Here's how the part is built. I have some questions about the finished solid (model axes, mm). A direction names the side the tool comes from. Give positions to 0.01 mm unless a question says otherwise; leave off trailing zeros. Order: outer loops, then holes, each group sorted by start corner. A loop starts at its lowest first (then second) coordinate and runs counter-clockwise, first axis right, second up.
from build123d import *

# Parameters (mm, degrees)
SKETCH_1_R      = 1.6
SKETCH_1_R_2    = 8
SKETCH_1_R_3    = 7.1
EXTRUDE_1_DEPTH = 5
SKETCH_1_3_R    = 7.1
SKETCH_1_3_R_2  = 2.1
EXTRUDE_2_DEPTH = 3
FILLET_1_R      = 1
FILLET_2_R      = 1
FILLET_3_R      = 1
FILLET_4_R      = 1


with BuildPart() as part:
    # Sketch 1 → Extrude 1 (new body)
    with BuildSketch(Plane(origin=(0, 0, 0), x_dir=(1, 0, 0), z_dir=(0, 1, 0))):
        with BuildLine():
            Line((1.92, -15.884382267), (51.2, -9.927738917))
            ThreePointArc((51.2, -9.927738917), (60, 0), (51.2, 9.927738917))
            Line((51.2, 9.927738917), (1.92, 15.884382267))
            ThreePointArc((1.92, 15.884382267), (-16, 0), (1.92, -15.884382267))
        make_face()
        with Locations((-12, 0)):
            Circle(SKETCH_1_R, mode=Mode.SUBTRACT)
        with Locations((0, 12)):
            Circle(SKETCH_1_R, mode=Mode.SUBTRACT)
        with Locations((12, 0)):
            Circle(SKETCH_1_R, mode=Mode.SUBTRACT)
        with Locations((0, -12)):
            Circle(SKETCH_1_R, mode=Mode.SUBTRACT)
        Circle(SKETCH_1_R_2, mode=Mode.SUBTRACT)
        with Locations((50, 0)):
            Circle(SKETCH_1_R_3, mode=Mode.SUBTRACT)
        Polygon((18.356508588, 8.861251331), (38.535462938, 6.422151611), (30.734984007, 2.266153232), align=None, mode=Mode.SUBTRACT)
        Polygon((18.356508588, -8.861251331), (38.535462938, -6.422151611), (30.734984007, -2.266153232), align=None, mode=Mode.SUBTRACT)
        with BuildLine():
            Line((14.72234722, 6.265180949), (26.481594346, 0))
            Line((26.481594346, 0), (14.72234722, -6.265180949))
            ThreePointArc((14.72234722, -6.265180949), (16, 0), (14.72234722, 6.265180949))
        make_face(mode=Mode.SUBTRACT)
        with BuildLine():
            Line((34.988373668, 0), (40.429404433, -2.898913674))
            ThreePointArc((40.429404433, -2.898913674), (40, 0), (40.429404433, 2.898913674))
            Line((40.429404433, 2.898913674), (34.988373668, 0))
        make_face(mode=Mode.SUBTRACT)
    extrude(amount=EXTRUDE_1_DEPTH)

    # Sketch 1_3 → Extrude 2 (add)
    with BuildSketch(Plane(origin=(0, 0, 0), x_dir=(1, 0, 0), z_dir=(0, 1, 0))):
        with Locations((50, 0)):
            Circle(SKETCH_1_3_R)
        with Locations((50, 0)):
            Circle(SKETCH_1_3_R_2, mode=Mode.SUBTRACT)
    extrude(amount=EXTRUDE_2_DEPTH)

    # Fillet 1
    fillet_1_edges = [part.edges().sort_by_distance(p)[0] for p in [
        (34.988373668, 2.5, 0),
        (40.429404433, 2.5, 2.898913674),
        (40.429404433, 2.5, -2.898913674),
    ]]
    fillet(fillet_1_edges, radius=FILLET_1_R)

    # Fillet 2
    fillet_2_edges = [part.edges().sort_by_distance(p)[0] for p in [
        (18.356508588, 2.5, 8.861251331),
        (38.535462938, 2.5, 6.422151611),
        (30.734984007, 2.5, 2.266153232),
    ]]
    fillet(fillet_2_edges, radius=FILLET_2_R)

    # Fillet 3
    fillet_3_edges = [part.edges().sort_by_distance(p)[0] for p in [
        (38.535462938, 2.5, -6.422151611),
        (18.356508588, 2.5, -8.861251331),
        (30.734984007, 2.5, -2.266153232),
    ]]
    fillet(fillet_3_edges, radius=FILLET_3_R)

    # Fillet 4
    fillet_4_edges = [part.edges().sort_by_distance(p)[0] for p in [
        (26.481594346, 2.5, 0),
        (14.72234722, 2.5, -6.265180949),
        (14.72234722, 2.5, 6.265180949),
    ]]
    fillet(fillet_4_edges, radius=FILLET_4_R)


solid = part.part
Q1. If we section it at C-C on x = 0: List the corners of the cut face in (y, z) for me, plus the area to 3 significant figures.
Filled sheet:
outline: (0, -16) - (5, -16) - (5, -13.6) - (0, -13.6) - close; (0, -10.4) - (5, -10.4) - (5, -8) - (0, -8) - close; (0, 8) - (5, 8) - (5, 10.4) - (0, 10.4) - close; (0, 13.6) - (5, 13.6) - (5, 16) - (0, 16) - close
area: 48.0 mm2
Q2. I'm going to push flat-ended pins straight in: P1, Ø13, axis at x = 50, z = 0, coming from the +Y side; P2, Ø3, axis at y = 0.5, z = -10, coming from the +X side; P3, Ø1, axis at y = 4.5, z = -1.5, coming from the -X side. Where does each tip first touch, or does it pass through?
Filled sheet:
P1: stops at y = 3
P2: stops at x = 55.27
P3: stops at x = -15.97
Q3. If we section it at D-D on x = 28.5: List the corners of the cut face in (y, z) for me, plus the area to 3 significant figures.
Filled sheet:
outline: (0, -12.67) - (5, -12.67) - (5, -7.64) - (0, -7.64) - close; (0, -3.46) - (5, -3.46) - (5, 3.46) - (0, 3.46) - close; (0, 7.64) - (5, 7.64) - (5, 12.67) - (0, 12.67) - close
area: 84.9 mm2
Q4. Thinking about a two-plate mould opening in Z: for faces 1 (the face through (26.215, 2.465, 12.948)), 2 (the face through (26.724, 2.465, -4.403)), 3 (the face through (60, 2, 0)), which applies, released by +Z, released by -Z, zero draft, split by the parting line, or undercut?
Filled sheet:
face 1: released by +Z
face 2: undercut
face 3: split by the parting line
Q5. If we section it at A-A on y = 0.75: Give the number of separate pieces and of enclosed holes in the cut face, plus the area to 3 significant figures.
Filled sheet:
separate pieces: 1
enclosed holes: 10
area: 1,460 mm2
Q6. I need wall thicknesses on L1, parallel to Z at x = 33, y = 1.2; L2, parallel to Y at x = 46, z = -4; L3, parallel to X at y = 1.95, z = 3.5. Which ranges of each line are inside material? Lowest first, please.
Filled sheet:
L1: z = -12.13 to -7.09, -3.47 to 3.47, 7.09 to 12.13
L2: y = 0 to 3
L3: x = -15.61 to -7.19, 7.19 to 15.61, 19.91 to 28.42, 33.05 to 59.37
Q7. For faces 4 (the face through (21.5, 0, 3.3)), 5 (the face through (29.44, 2.46, -7.52)), 6 (the face through (51.5, 3, -1.7)), which set-ups out of +Z, -Z, +X, -X, +Y, -Y let a thin tool reach every point of the face, with its end or its side?
Filled sheet:
face 4: +Z, -Z, +X, -X, -Y
face 5: +Y, -Y
face 6: +Y
